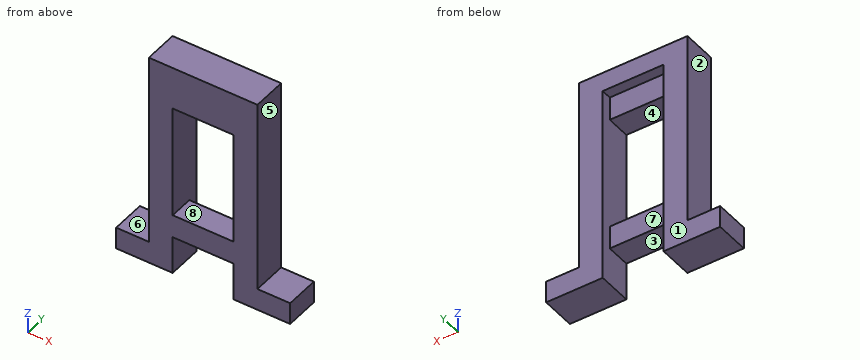
```python
from build123d import *

# Parameters (mm, degrees)
F0_W     = 12.6
F0_H     = 23.4
F1_DEPTH = 7.1
F2_W     = 12.6
F2_H     = 4.8
F2_H_2   = 4.88
F3_DEPTH = 2.12


with BuildPart() as f1:
    # F0 (on Front) → F1 (new body)
    with BuildSketch(Plane.XZ):
        Polygon((11.23, 22.465), (-11.23, 22.465), (-11.23, -17.915), (-17.99, -17.915), (-17.99, -22.465), (-6.3, -22.465), (-6.3, -14.615), (6.3, -14.615), (6.3, -22.465), (17.99, -22.465), (17.99, -17.915), (11.23, -17.915), align=None)
        with Locations((0, 1.885)):
            Rectangle(F0_W, F0_H, mode=Mode.SUBTRACT)
    extrude(amount=F1_DEPTH)

    # F2 (on face) → F3 (cut)
    with BuildSketch(Plane(origin=(0, 0, 0), x_dir=(-1, 0, 0), z_dir=(0, 1, 0))):
        with Locations((0, -12.215)):
            Rectangle(F2_W, F2_H)
        with Locations((0, 16.025)):
            Rectangle(F2_W, F2_H_2)
    extrude(amount=-F3_DEPTH, mode=Mode.SUBTRACT)


solid = f1.part
```
Part model, mm, in its own coordinate system. Face numbers are marked on the shaded views. A direction names the side the tool comes from. Round coordinates to 2 decimals unless told otherwise and drop trailing zeros. Order: outer loops, then holes, each group sorted by start corner. A loop starts at its lowest first (then second) coordinate and runs counter-clockwise, first axis right, second up. Notation, with made-up numbers: M 37,77.25 L 58,77.25 A6 ccw 58,84.25 Z; hole C 83.25,22 d9. An arc over 180 degrees is marked long. Answer in a Markdown table with one row per item. Add a question column.
Q1. Cut at C-C on z = -6.5. Give the cut face in (x, y).
Q2. Cut at B-B on y = -5.5. Give the cut face in (x, z) (3 decimals), and give its area (3 significant figures).
Q3. Cut at A-A on x = -2. Give the cut face in (y, z) (3 decimals).
Q4. 3-axis set-ups, long thin cutter, end or side, ignore diameter. For the marked faces 5, 6, 7 and 8: which of +Z, -Z, +X, -X, +Y, -Y reach the whole face in a straight line?
Q5. Mould opens along X. For the marked faces 1, 2, 3 and 4 say: +X half, -X half, draft (parallel to the pull), parting line (faces both ways), or undercut.
Q6. Pin check, flat tips, straight feed: pin 1 (0.6 mm diameter, centred on x = -2, y = -0.5, fed in from -Z) (3 decimals); pin 2 (3.5 mm diameter, centred on y = -4.5, z = 5, fed in from +X); pin 3 (3 mm diameter, centred on y = -3, z = -4.5, fed in from -X). Stop position of each tip, or through.
Q7. Wall check: L1, parallel to X at y = -4.25, z = -18.5; L2, parallel to X at y = -4, z = -9; L3, parallel to Z at x = 2, y = -2.25 (3 decimals). Give the ranges that are in metal, low to high. Write a range as from..to.
Q8. Cut at D-D on y = -0.5. Give the cut face in (x, z) (3 decimals).
Established:
| question | item | result |
|---|---|---|
| 1 | outline | M -11.23,-7.1 L -6.3,-7.1 L -6.3,0 L -11.23,0 Z; M 6.3,-7.1 L 11.23,-7.1 L 11.23,0 L 6.3,0 Z |
| 2 | outline | M -17.99,-22.465 L -6.3,-22.465 L -6.3,-14.615 L 6.3,-14.615 L 6.3,-22.465 L 17.99,-22.465 L 17.99,-17.915 L 11.23,-17.915 L 11.23,22.465 L -11.23,22.465 L -11.23,-17.915 L -17.99,-17.915 Z; hole M -6.3,-9.815 L 6.3,-9.815 L 6.3,13.585 L -6.3,13.585 Z |
| 2 | area | 677 mm2 |
| 3 | outline | M -7.1,-14.615 L -2.12,-14.615 L -2.12,-9.815 L -7.1,-9.815 Z; M -7.1,13.585 L -2.12,13.585 L -2.12,18.465 L 0,18.465 L 0,22.465 L -7.1,22.465 Z |
| 4 | face 5 | +Z, +X, +Y, -Y |
| 4 | face 6 | +Z, -X, +Y, -Y |
| 4 | face 7 | -Z, +Y |
| 4 | face 8 | +Y, -Y |
| 5 | face 1 | draft |
| 5 | face 2 | -X half |
| 5 | face 3 | undercut |
| 5 | face 4 | undercut |
| 6 | pin 1 | stops at z = 18.465 |
| 6 | pin 2 | stops at x = 11.23 |
| 6 | pin 3 | stops at x = -11.23 |
| 7 | L1 | x = -17.99..-6.3, 6.3..17.99 |
| 7 | L2 | x = -11.23..-6.3, 6.3..11.23 |
| 7 | L3 | z = -14.615..-9.815, 13.585..22.465 |
| 8 | outline | M -17.99,-22.465 L -6.3,-22.465 L -6.3,18.465 L 6.3,18.465 L 6.3,-22.465 L 17.99,-22.465 L 17.99,-17.915 L 11.23,-17.915 L 11.23,22.465 L -11.23,22.465 L -11.23,-17.915 L -17.99,-17.915 Z |
